Geometry check sheet. Reference: the model listing, model coordinates, mm. A direction names the side the tool comes from. Round coordinates to 2 decimals unless told otherwise and drop trailing zeros. Write each loop counter-clockwise with the first axis right and the second up, starting at its lowest first coordinate (ties: lowest second). Pieces come first, ordered by that corner, then holes. Notation, with made-up numbers: M 63.25,24 L 68.25,24 A11 ccw 68.25,36 Z; hole C 42.5,14 d6. An arc over 180 degrees is marked long. Put each result on its own line as item: value. Start each with the question number.
(1) Section check C-C on y = 12.5. Record the cut outline in (x, z), then the cut area to 3 significant figures.
(2) Section check D-D on x = 134.5. Record the cut outline in (y, z).
(3) Section check B-B on z = 25.5. Record the cut outline in (x, y), then the cut area to 3 significant figures.
(4) Section check A-A on x = 76. Record the cut outline in (y, z), then the cut area to 3 significant figures.
(5) Mould release check, pull along X, two halves, no side actions. Record for faces 1 (the flat face through (92.4, 84, 21)), 2 (the flat face through (125, 101.6, 42)), 3 (the flat face through (74, 42, 1.2)): pulls with the +X half, pulls with the -X half, needs draft (parallel to the pull), parting line crosses it, or undercut.
(6) Tool access check on faces 4 (the flat face through (129.843, 23.116, 20.92)), 5 (the flat face through (149.52, 73, 21)), 6 (the flat face through (56, 2.88, 21)), 7 (the flat face through (44, 60, 21)), 8 (the flat face through (74, 42, 41.2)). Record the directions out of +Z, -Z, +X, -X, +Y, -Y that give a thin tool (end or side, any length) a straight path to the whole face; none if there is none.
(7) Material ranges on probe 1 along Y at (x, z) = (33.5, 20.5); probe 2 along Z at (x, y) = (92.5, 17); probe 3 along X at (y, z) = (96.5, 11), recorded low to high.
(8) Gauge pin test, flat ends, axial feed: pin 1 (12 mm diameter, centred on x = 47, z = 28, fed in from +Y); pin 2 (1.5 mm diameter, centred on y = 30.5, z = 11, fed in from -X); pin 3 (4 mm diameter, centred on y = 39, z = 11.5, fed in from -X). Record the tip position at first contact, or that the pin passes through.
from build123d import *

# Parameters (mm, degrees)
F1_DEPTH = 1.2
F4_DEPTH = 40
F6_DEPTH = 1.2


with BuildPart() as f1:
    # F0 (on Top) → F1 (new body)
    with BuildSketch(Plane.XY):
        Polygon((0, 60), (0, 0), (110.8, 0), (152.4, 41.6), (152.4, 101.6), (92.4, 101.6), (92.4, 66.452814), (85.947186, 60), align=None)
    extrude(amount=F1_DEPTH)

    # F2 (on face) + F3 (on face) → F4 (join)
    with BuildSketch(Plane.XY.offset(1.2)):
        Polygon((109.607065, 2.88), (0, 2.88), (0, 0), (110.8, 0), (152.4, 41.6), (152.4, 101.6), (149.52, 101.6), (149.52, 42.792935), align=None)
    with BuildSketch(Plane.XY.offset(1.2)):
        Polygon((85.947186, 60), (0, 60), (0, 57.12), (87.140121, 57.12), (95.28, 65.259879), (95.28, 101.6), (92.4, 101.6), (92.4, 66.452814), align=None)
    extrude(amount=F4_DEPTH)

    # F5 (on face) → F6 (join)
    with BuildSketch(Plane.XY.offset(41.2)):
        Polygon((92.4, 66.452814), (85.947186, 60), (0, 60), (0, 0), (110.8, 0), (152.4, 41.6), (152.4, 101.6), (92.4, 101.6), align=None)
    extrude(amount=F6_DEPTH)


solid = f1.part
Answers follow:
1. outline: M 0,0 L 123.3,0 L 123.3,42.4 L 0,42.4 L 0,41.2 L 119.23,41.2 L 119.23,1.2 L 0,1.2 Z
1. area: 459 mm^2
2. outline: M 23.7,0 L 101.6,0 L 101.6,1.2 L 27.77,1.2 L 27.77,41.2 L 101.6,41.2 L 101.6,42.4 L 23.7,42.4 Z
3. outline: M 0,0 L 110.8,0 L 152.4,41.6 L 152.4,101.6 L 149.52,101.6 L 149.52,42.79 L 109.61,2.88 L 0,2.88 Z; M 0,57.12 L 87.14,57.12 L 95.28,65.26 L 95.28,101.6 L 92.4,101.6 L 92.4,66.45 L 85.95,60 L 0,60 Z
3. area: 1,040 mm^2
4. outline: M 0,0 L 60,0 L 60,42.4 L 0,42.4 Z; hole M 2.88,1.2 L 57.12,1.2 L 57.12,41.2 L 2.88,41.2 Z
4. area: 374 mm^2
5. face 1: pulls with the -X half
5. face 2: needs draft
5. face 3: undercut
6. face 4: -X, +Y
6. face 5: +Y
6. face 6: -X
6. face 7: +Z, -Z, -X, +Y
6. face 8: none
7. probe 1: y = 0 to 2.88, 57.12 to 60
7. probe 2: z = 0 to 1.2, 41.2 to 42.4
7. probe 3: x = 92.4 to 95.28, 149.52 to 152.4
8. pin 1: stops at y = 60
8. pin 2: stops at x = 136.48
8. pin 3: stops at x = 143.73
